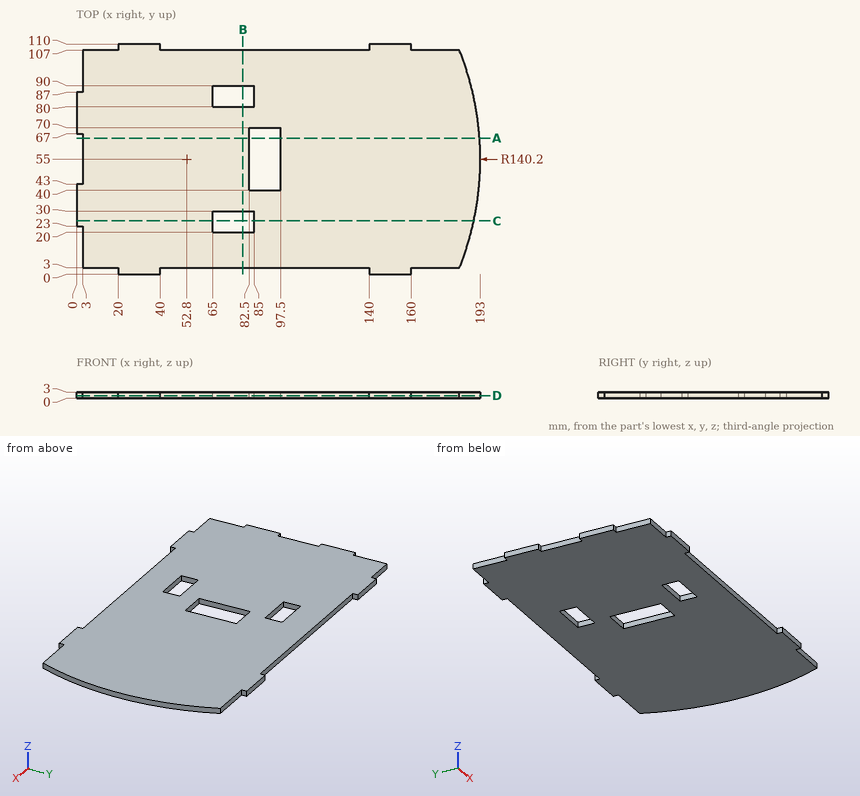
Print and shaded views of the part. All mm, measured from the part's lowest x, y and z. Give positions to 0.01 mm unless a question says otherwise; leave off trailing zeros. Loops run counter-clockwise (first coordinate to the right, second up) from the corner with the lowest first, then second, coordinate; pieces in that order, holes last. Notation, with made-up numbers: (-11.5, 14.25) - (46.5, 14.25) arc R28 cw to (46.5, 50.25) - close; hole circle Ø5 at (58.5, -26). An arc over 180 degrees is marked (long way). One line per item, written item: value. Start each with the question number.
1. Slice it at A-A (y = 65). List the corners of the cut face in (x, z), plus the area to 3 significant figures.
2. Slice it at C-C (y = 25.5). List the corners of the cut face in (x, z).
3. Probe L1, parallel to Y at x = 89, z = 2.1; L2, parallel to Y at x = 112, z = 1.25; L3, parallel to X at y = 43.5, z = 1.4. List the from-to ranges inside material, lowest first. Write a range as from..to.
4. Slice it at D-D (z = 1.3). Give the number of separate pieces and of enclosed holes in the cut face, plus the area to 3 significant figures.
5. Slice it at B-B (x = 79.5). List the corners of the cut face in (y, z), plus the area to 3 significant figures.
6. Pin check, flat tips, straight feed: pin 1 (0.9 mm diameter, centred on y = 2, z = 1.5, fed in from -X); pin 2 (1.5 mm diameter, centred on y = 78, z = 0.5, fed in from -X); pin 3 (0.9 mm diameter, centred on x = 95.5, z = 2, fed in from +Y); pin 4 (1.5 mm diameter, centred on x = 2, z = 1.5, fed in from -Y). Stop position of each tip, or through.
Solution:
1. outline: (3, 0) - (82.5, 0) - (82.5, 3) - (3, 3) - close; (97.5, 0) - (192.64, 0) - (192.64, 3) - (97.5, 3) - close
1. area: 524 mm^2
2. outline: (0, 0) - (65, 0) - (65, 3) - (0, 3) - close; (85, 0) - (189.86, 0) - (189.86, 3) - (85, 3) - close
3. L1: y = 3..40, 70..107
3. L2: y = 3..107
3. L3: x = 3..82.5, 97.5..192.53
4. separate pieces: 1
4. enclosed holes: 3
4. area: 18,900 mm^2
5. outline: (3, 0) - (20, 0) - (20, 3) - (3, 3) - close; (30, 0) - (80, 0) - (80, 3) - (30, 3) - close; (90, 0) - (107, 0) - (107, 3) - (90, 3) - close
5. area: 252 mm^2
6. pin 1: stops at x = 20
6. pin 2: stops at x = 0
6. pin 3: stops at y = 107
6. pin 4: stops at y = 23
